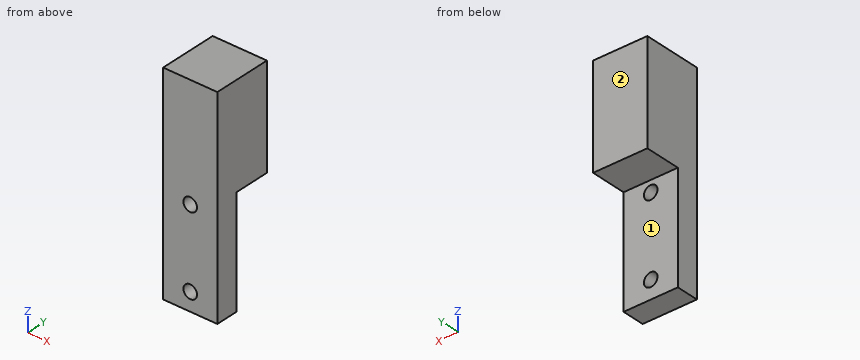
from build123d import *

# Parameters (mm, degrees)
SKETCH1_W           = 12
SKETCH1_H           = 46.47
SKETCH1_R           = 1.5
BOSS_EXTRUDE1_DEPTH = 5
SKETCH2_W           = 12
SKETCH2_H           = 22.5
BOSS_EXTRUDE2_DEPTH = 8


with BuildPart() as part:
    # Sketch1 → Boss-Extrude1 (new body)
    with BuildSketch(Plane(origin=(0, 0, 0), x_dir=(1, 0, 0), z_dir=(0, 1, 0))):
        Rectangle(SKETCH1_W, SKETCH1_H)
        with Locations(Location((0, 19.235, 0), (0, 0, 270))):
            Circle(SKETCH1_R, mode=Mode.SUBTRACT)
        with Locations(Location((0, 1.765, 0), (0, 0, 270))):
            Circle(SKETCH1_R, mode=Mode.SUBTRACT)
    extrude(amount=-BOSS_EXTRUDE1_DEPTH)

    # Sketch2 → Boss-Extrude2 (add)
    with BuildSketch(Plane(origin=(0, 0, 0), x_dir=(1, 0, 0), z_dir=(0, 1, 0))):
        with Locations((0, -11.985)):
            Rectangle(SKETCH2_W, SKETCH2_H)
    extrude(amount=BOSS_EXTRUDE2_DEPTH)


solid = part.part
Input: part model. Units: mm. Frame: model coordinates. Face numbers are marked on the shaded views. A direction names the side the tool comes from. Round coordinates to 2 decimals unless told otherwise and drop trailing zeros. Order: outer loops, then holes, each group sorted by start corner. A loop starts at its lowest first (then second) coordinate and runs counter-clockwise, first axis right, second up. Notation, with made-up numbers: (38, 67) - (57, 67) arc R20 cw to (57, 93) - close; hole circle Ø5 at (28, 49). An arc over 180 degrees is marked (long way). Answer as a JSON object with one key per item and string values. Group by question number.
(1) Cut plane D-D (x = 4). Return loops of the section in (y, z) (3 decimals).
(2) Cut plane B-B (z = -20). Return loops of the section in (x, y).
(3) Pin query (flat end, axial travel): P1, Ø2.5, axis at x = -2.5, y = 2.5, coming from the -Z side (3 decimals); P2, Ø6, axis at y = 2, z = -12, coming from the -X side; P3, Ø6, axis at x = -3, z = -7.5, coming from the +Y side; P4, Ø2.5, axis at x = 0, z = -19.235, coming from the -Y side. Return the tip coordinate at first contact, or that it passes through.
(4) Cut plane A-A (x = 0). Return loops of the section in (y, z) (3 decimals).
(5) Reachability of the marked faces 1 and 2 from +Z, -Z, +X, -X, +Y, -Y: full face, straight path, thin tool, end or side. Return the list, or none.
(6) Material intervals for probe 1 along Z at (x, y) = (2.25, 7.5) (3 decimals); probe 2 along Y at (x, z) = (-2.5, -2); probe 3 along X at (y, z) = (-1.25, -2.5), sorted ascending. Write a range as from..to.
(7) Cut plane C-C (y = -1.75). Return loops of the section in (x, z) (3 decimals), then the cut area to 3 significant figures.
Here are the results:
{
 "1": {"outline": "(-5, -23.235) - (0, -23.235) - (0, 0.735) - (8, 0.735) - (8, 23.235) - (-5, 23.235) - close"},
 "2": {"outline": "(-6, -5) - (-1.29, -5) - (-1.29, 0) - (-6, 0) - close; (1.29, -5) - (6, -5) - (6, 0) - (1.29, 0) - close"},
 "3": {"P1": "stops at z = 0.735", "P2": "stops at x = -6", "P3": "stops at y = 0", "P4": "passes through"},
 "4": {"outline": "(-5, -23.235) - (0, -23.235) - (0, -20.735) - (-5, -20.735) - close; (-5, -17.735) - (0, -17.735) - (0, -3.265) - (-5, -3.265) - close; (-5, -0.265) - (0, -0.265) - (0, 0.735) - (8, 0.735) - (8, 23.235) - (-5, 23.235) - close"},
 "5": {"face 1": "-Z, +X, -X, +Y", "face 2": "+Z, -Z, +X, -X, +Y"},
 "6": {"probe 1": "z = 0.735..23.235", "probe 2": "y = -5..0", "probe 3": "x = -6..-1.31, 1.31..6"},
 "7": {"outline": "(-6, -23.235) - (6, -23.235) - (6, 23.235) - (-6, 23.235) - close; hole circle Ø3 at (0, -19.235); hole circle Ø3 at (0, -1.765)", "area": "544 mm^2"}
}
